```python
from build123d import *

# Parameters (mm, degrees)
BOSS_EXTRUDE1_DEPTH = 12.5
SKETCH6_W           = 9
SKETCH6_H           = 9
CUT_EXTRUDE2_DEPTH  = 19


with BuildPart() as part:
    # Sketch3 → Boss-Extrude1 (new body)
    with BuildSketch(Plane.XY):
        Polygon((51.444398057, 20.442826613), (25.886157296, 20.442826613), (25.886157296, -19.557173387), (51.444398057, -19.557173387), (51.444398057, -12.557173387), (34.444398057, -12.557173387), (34.444398057, 10.442826613), (51.444398057, 10.442826613), align=None)
    extrude(amount=BOSS_EXTRUDE1_DEPTH)

    # Sketch6 → Cut-Extrude2 (cut)
    with BuildSketch(Plane.ZY.offset(-25.886157296)):
        with Locations((6.342638548, -13.057173387)):
            Rectangle(SKETCH6_W, SKETCH6_H)
    extrude(amount=-CUT_EXTRUDE2_DEPTH, mode=Mode.SUBTRACT)


solid = part.part
```
Work out the finished part from the listing and answer in its coordinate system (mm). A direction names the side the tool comes from. Coordinates: 2 decimals unless noted, no trailing zeros. Write each loop counter-clockwise with the first axis right and the second up, starting at its lowest first coordinate (ties: lowest second). Pieces come first, ordered by that corner, then holes.
Q1. A cutting plane is placed at A-A, the plane y = -11. Give the vertices of the cut face in (x, z).
Q2. Find the intervals of material crossed by line 1 (Y direction, x = 45, z = 8); line 2 (Y direction, x = 43.25, z = 4); line 3 (Z direction, x = 43.5, y = -17), in increasing order.
Q3. A cutting plane is placed at B-B, the plane x = 49. Give the vertices of the cut face in (y, z).
Q4. Determine the mould class of faces 1 (the face through (39, 20.443, 6)), 2 (the face through (51.444, 15, 6)), 3 (the face through (33, -14, 10.843)), 4 (the face through (38, -19.557, 6)) for opening direction Y: released by +Y, released by -Y, zero draft, split by the parting line, or undercut.
Q5. Which of the six approach directions +Z, -Z, +X, -X, +Y, -Y give full straight-line access (tool end or side, diameter ignored) to faces 5 (the face through (47, -12.557, 6)), 6 (the face through (25.886, 5, 6)), 7 (the face through (30, -8.557, 6)), 8 (the face through (35, -17.557, 6))?
Q6. A cutting plane is placed at D-D, the plane x = 29.5. Give the vertices of the cut face in (y, z), then the cut area to 3 significant figures.
Q7. This flat-tipped pin is pushed along its axis until it touches: pin 1 Ø2 at (x, y) = (37, 7) entering from -Z. Where does it stop, or does it pass through?
Q8. A cutting plane is placed at C-C, the plane z = 3.5. Give the vertices of the cut face in (x, y).
Findings below:
1. outline: (25.89, 0) - (34.44, 0) - (34.44, 1.84) - (25.89, 1.84) - close; (25.89, 10.84) - (34.44, 10.84) - (34.44, 12.5) - (25.89, 12.5) - close
2. line 1: y = -19.56 to -12.56, 10.44 to 20.44
2. line 2: y = -19.56 to -17.56, 10.44 to 20.44
2. line 3: z = 0 to 1.84, 10.84 to 12.5
3. outline: (-19.56, 0) - (-12.56, 0) - (-12.56, 12.5) - (-19.56, 12.5) - close; (10.44, 0) - (20.44, 0) - (20.44, 12.5) - (10.44, 12.5) - close
4. face 1: released by +Y
4. face 2: zero draft
4. face 3: undercut
4. face 4: released by -Y
5. face 5: +Z, -Z, +X
5. face 6: +Z, -Z, -X, +Y, -Y
5. face 7: +X, -X
5. face 8: -X
6. outline: (-19.56, 0) - (20.44, 0) - (20.44, 12.5) - (-19.56, 12.5) - close; hole (-17.56, 1.84) - (-8.56, 1.84) - (-8.56, 10.84) - (-17.56, 10.84) - close
6. area: 419 mm2
7. pin 1: passes through
8. outline: (25.89, -19.56) - (51.44, -19.56) - (51.44, -12.56) - (44.89, -12.56) - (44.89, -17.56) - (25.89, -17.56) - close; (25.89, -8.56) - (34.44, -8.56) - (34.44, 10.44) - (51.44, 10.44) - (51.44, 20.44) - (25.89, 20.44) - close
